Job drawing, mm, ordinate dimensions from the low corner. One solid piece. Coordinates: 2 decimals unless noted, no trailing zeros. Order: outer loops, then holes, each group sorted by start corner. A loop starts at its lowest first (then second) coordinate and runs counter-clockwise, first axis right, second up. Notation, with made-up numbers: (-1.5, 88) - (13.5, 88) arc R17 ccw to (13.5, 112) - close; hole circle Ø7 at (5.25, -11). An arc over 180 degrees is marked (long way). Return JSON: item names as keys, results as strings.
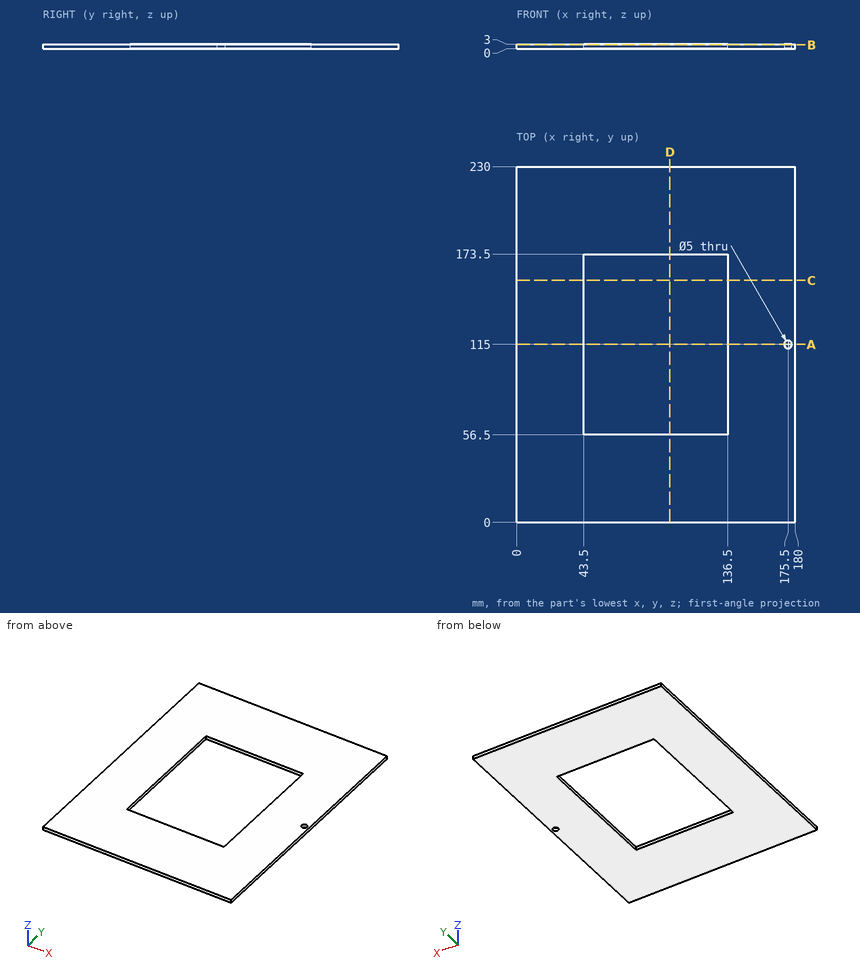
1. Drop a flat-ended pin along its axis: pin 1 (1.5 mm diameter, centred on y = 109.5, z = 2, fed in from -X). Give the stop position or say it passes through.
Check values:
{"pin 1": "x = 0"}
2. Probe L1, parallel to X at y = 115, z = 1.9; L2, parallel to X at y = 168, z = 2; L3, parallel to Y at x = 175.5, z = 1.7. List the from-to ranges inside material, lowest first.
Check values:
{"L1": "0 to 43.5, 136.5 to 173, 178 to 180", "L2": "0 to 43.5, 136.5 to 180", "L3": "0 to 112.5, 117.5 to 230"}
3. Cut at D-D on x = 99. Give the cut face in (y, z), plus the area to 3 significant figures.
Check values:
{"outline": "(0, 0) - (56.5, 0) - (56.5, 3) - (0, 3) - close; (173.5, 0) - (230, 0) - (230, 3) - (173.5, 3) - close", "area": "339 mm²"}
4. Cut at C-C on y = 156.5. Give the cut face in (x, z).
Check values:
{"outline": "(0, 0) - (43.5, 0) - (43.5, 3) - (0, 3) - close; (136.5, 0) - (180, 0) - (180, 3) - (136.5, 3) - close"}
5. Cut at B-B on z = 2.5. Give the cut face in (x, y), plus the area to 3 significant figures.
Check values:
{"outline": "(0, 0) - (180, 0) - (180, 230) - (0, 230) - close; hole (43.5, 56.5) - (136.5, 56.5) - (136.5, 173.5) - (43.5, 173.5) - close; hole circle Ø5 at (175.5, 115)", "area": "30,500 mm²"}
6. Cut at A-A on y = 115. Give the cut face in (x, z).
Check values:
{"outline": "(0, 0) - (43.5, 0) - (43.5, 3) - (0, 3) - close; (136.5, 0) - (173, 0) - (173, 3) - (136.5, 3) - close; (178, 0) - (180, 0) - (180, 3) - (178, 3) - close"}
